Input: part model. Units: mm. Frame: model coordinates. A direction names the side the tool comes from. Give positions to 0.01 mm unless a question says otherwise; leave off trailing zeros. Loops run counter-clockwise (first coordinate to the right, second up) from the corner with the lowest first, then second, coordinate; pieces in that order, holes last. Notation, with made-up numbers: (16, -2.5) -> (42, -2.5) arc R17 cw to (42, 15.5) -> close; hole circle Ø4 at (64, -24.5). An arc over 180 degrees is marked (long way). Answer as a JSON object with one key per item and string values. Group by question number.
```python
from build123d import *

# Parameters (mm, degrees)
F1_DEPTH = 199.5424
F2_SIZE  = 22.352
F3_R     = 2.4638
F4_DEPTH = 25.4


with BuildPart() as f1:
    # F0 (on Top) → F1 (new body)
    with BuildSketch(Plane.XY):
        with BuildLine():
            Line((0, -31.75), (0, -7.0612))
            ThreePointArc((0, -7.0612), (-2.068178, -2.068178), (-7.0612, 0))
            Line((-7.0612, 0), (-31.75, 0))
            Line((-31.75, 0), (-31.75, -4.7752))
            Line((-31.75, -4.7752), (-7.0612, -4.7752))
            ThreePointArc((-7.0612, -4.7752), (-5.444754, -5.444754), (-4.7752, -7.0612))
            Line((-4.7752, -7.0612), (-4.7752, -31.75))
            Line((-4.7752, -31.75), (0, -31.75))
        make_face()
    extrude(amount=F1_DEPTH)

    # F2
    f2_edges = [f1.edges().sort_by_distance(p)[0] for p in [
        (-2.3876, -31.75, 199.5424),
        (-2.3876, -31.75, 0),
    ]]
    chamfer(f2_edges, length=F2_SIZE)

    # F3 (on Front) → F4 (cut)
    with BuildSketch(Plane.XZ):
        with Locations((-20.193, 174.1424)):
            Circle(F3_R)
        with Locations((-20.193, 99.7712)):
            Circle(F3_R)
        with Locations((-20.193, 25.4)):
            Circle(F3_R)
        with Locations((-20.193, 147.3962)):
            Circle(F3_R)
        with Locations((-20.193, 52.1462)):
            Circle(F3_R)
    extrude(amount=F4_DEPTH, mode=Mode.SUBTRACT)


solid = f1.part
```
Q1. Section A-A on z = 25.4. Return the cut outline in (x, y).
Q2. Pull-direction query (Z, two-part tool) for faces 1 (the face through (-20.51, -2.35, 149.84)), 2 (the face through (-17, -4.775, 98)), 3 (the face through (-2.42, -20.42, 188.52)); classes: +Z half, -Z half, draft (parallel to the pull), parting line (faces both ways), or undercut.
Q3. Section B-B on x = -15. Return the cut outline in (y, z), then the cut area to 3 significant figures.
Q4. Section C-C on y = -29. Return the cut outline in (x, z).
Q5. Set-up query: faces 4 (the face through (-16, 0, 98)), 5 (the face through (-4.775, -19, 98)). Return all of +Z, -Z, +X, -X, +Y, -Y with unobstructed straight access to the full face (end or side cutting, diameter ignored); none if empty.
Q6. Pin query (flat end, axial travel): pin 1 Ø6.5 at (x, z) = (-20.193, 25.4) entering from -Y; pin 2 Ø1 at (y, z) = (-20.5, 146.5) entering from -X. Return the tip coordinate at first contact, or that it passes through.
Q7. Ray query, probe 1 along Y at (x, z) = (-26.5, 172); probe 2 along Y at (x, z) = (-5, 109). Return the intervals inside material, ascending.
Numbers:
{
 "1": {"outline": "(-31.75, -4.78) -> (-22.66, -4.78) -> (-22.66, 0) -> (-31.75, 0) -> close; (-17.73, -4.78) -> (-7.06, -4.78) arc R2.29 cw to (-4.78, -7.06) -> (-4.78, -31.75) -> (0, -31.75) -> (0, -7.06) arc R7.06 ccw to (-7.06, 0) -> (-17.73, 0) -> close"},
 "2": {"face 1": "undercut", "face 2": "draft", "face 3": "+Z half"},
 "3": {"outline": "(-4.78, 0) -> (0, 0) -> (0, 199.54) -> (-4.78, 199.54) -> close", "area": "953 mm²"},
 "4": {"outline": "(-4.78, 19.6) -> (0, 19.6) -> (0, 179.94) -> (-4.78, 179.94) -> close"},
 "5": {"face 4": "+Z, -Z, +X, -X, +Y", "face 5": "+Z, -Z, -X, -Y"},
 "6": {"pin 1": "stops at y = -4.78", "pin 2": "stops at x = -4.78"},
 "7": {"probe 1": "y = -4.78 to 0", "probe 2": "y = -6.07 to -0.31"}
}
